Autodesk Inventor part; units mm, degrees
ref_plane "YZ Plane" through (0, 0, 0) normal (1, 0, 0) x (0, 1, 0)
ref_plane "XZ Plane" through (0, 0, 0) normal (0, 1, 0) x (-1, 0, 0)
ref_plane "XY Plane" through (0, 0, 0) normal (0, 0, 1) x (1, 0, 0)
sketch "Boceto1" plane through (0, 0, 0) normal (0, 0, 1) x (1, 0, 0)
  circle A0 centre (0, 0) radius 80
  dimension "d0" = 160
extrude "Extrusión1" add sketch "Boceto1" against normal blind 542
sketch "Boceto2" plane through (0, 0, 0) normal (0, 0, 1) x (1, 0, 0)
  line L0 (-70, 80) -> (70, 80)
  line L1 (80, 70) -> (80, -70)
  line L2 (70, -80) -> (-70, -80)
  line L3 (-80, -70) -> (-80, 70)
  circle A0 centre (0, 0) radius 80 construction
  circle A1 centre (-70, 70) radius 3
  arc A2 (-70, 80) -> (-80, 70) centre (-70, 70) ccw
  arc A3 (80, 70) -> (70, 80) centre (70, 70) ccw
  arc A4 (70, -80) -> (80, -70) centre (70, -70) ccw
  arc A5 (-80, -70) -> (-70, -80) centre (-70, -70) ccw
  circle A6 centre (-70, -70) radius 3
  circle A7 centre (70, -70) radius 3
  circle A8 centre (70, 70) radius 3
  dimension "d4" = 6
  dimension "d5" = 10
  dimension "d6" = 10
  dimension "d7" = 10
  dimension "d10" = 360
extrude "Extrusión2" add sketch "Boceto2" along normal blind 10
sketch "Boceto3" plane through (0, 0, 10) normal (0, 0, 1) x (1, 0, 0)
  circle A0 centre (0, 0) radius 58.4375 construction
  circle A1 centre (0, 58.4375) radius 20.625
  circle A2 centre (0, 0) radius 58.4375 construction
  circle A3 centre (-55.5774, 18.0582) radius 20.625
  circle A4 centre (0, 0) radius 58.4375 construction
  circle A5 centre (-34.3487, -47.2769) radius 20.625
  circle A6 centre (0, 0) radius 58.4375 construction
  circle A7 centre (34.3487, -47.2769) radius 20.625
  circle A8 centre (0, 0) radius 58.4375 construction
  circle A9 centre (55.5774, 18.0582) radius 20.625
  dimension "d14" = 116.875
  dimension "d15" = 41.25
  dimension "d18" = 360
extrude "Extrusión3" add sketch "Boceto3" along normal blind 472.3
equation "\"d1\" = 2 * ancho_llanta"
equation "\"d6\" = d5"
equation "\"ancho_llanta\" = 271"
properties part number "atornillador" material "Acero inoxidable, pulido"
Could you check a few things on this model? Use its own coordinates, in mm. A direction names the side the tool comes from. Round coordinates to 2 decimals unless told otherwise and drop trailing zeros.
(1) Suppose I cut it at A-A on z = 413. State how many separate pieces and enclosed holes the cut face has, and give its area (3 significant figures).
Findings below:
separate pieces: 5
enclosed holes: 0
area: 6,680 mm2
(2) For pin 1 (2 mm diameter, centred on x = -10.5, z = 289.5, fed in from +Y); pin 2 (4 mm diameter, centred on y = -53, z = -416.5, fed in from +X); pin 3 (4 mm diameter, centred on x = 52.5, z = -406.5, fed in from +Y), each with a flat end and sliding along its axis, tell me the tip position at first contact or that it passes through.
Findings below:
pin 1: stops at y = 76.74
pin 2: stops at x = 61.64
pin 3: stops at y = 62.05
(3) Thinking about a two-plate mould opening in Y: for faces 1 (the face through (61, 61, 0)), 2 (the face through (-17.34, -78.1, -267.21)), 3 (the face through (40.376, 4.119, 242.844)), which applies, +Y half, -Y half, draft (parallel to the pull), parting line (faces both ways), or undercut?
Findings below:
face 1: draft
face 2: parting line
face 3: undercut
(4) If I drill on probe 1 along Y at (x, z) = (70, 4.5); probe 2 along Z at (x, y) = (-50, -71); probe 3 along Z at (x, y) = (-39.5, 49.5), over which ranges is the centre line in solid material (lowest first)?
Findings below:
probe 1: y = -80 to -73, -67 to 67, 73 to 80
probe 2: z = 0 to 10
probe 3: z = -542 to 10
(5) Which directions (+Z, -Z, +X, -X, +Y, -Y) give clear straight access to the entire face, cutting with the end or side of a thin tool? Please do faces 4 (the face through (-61, 64, 0)), 5 (the face through (-61, -61, 0)), 6 (the face through (-16.367, 70.987, 242.844)), 7 (the face through (61, -64, 0)), 8 (the face through (55, 18, 482.3)).
Findings below:
face 4: -Z, -X, +Y
face 5: -Z, -X, -Y
face 6: +Z
face 7: -Z, +X, -Y
face 8: +Z, +X, -X, +Y, -Y
